```python
from build123d import *

# Parameters (mm, degrees)
SKETCH1_R               = 40
BOSS_EXTRUDE1_DEPTH     = 31.5
CUT_EXTRUDE1_DEPTH      = 65.747586828
CUT_EXTRUDE1_DEPTH_BACK = 65.747586828
SKETCH2_R               = 3
SKETCH7_R               = 10
CUT_EXTRUDE3_DEPTH      = 21
SKETCH8_R               = 6.5
CUT_EXTRUDE4_DEPTH      = 8
SKETCH9_R               = 7.5
CUT_EXTRUDE5_DEPTH      = 6
SKETCH10_R              = 2
CUT_EXTRUDE7_DEPTH      = 65.747587
CIRPATTERN1_COUNT       = 4
SKETCH12_R              = 4
CUT_EXTRUDE8_DEPTH      = 4
CIRPATTERN2_COUNT       = 4
FILLET1_R               = 4


with BuildPart() as part:
    # Sketch1 → Boss-Extrude1 (new body)
    with BuildSketch(Plane(origin=(0, 0, 0), x_dir=(1, 0, 0), z_dir=(0, 1, 0))):
        with Locations(Location((0, 0, 0), (0, 0, 270))):
            Circle(SKETCH1_R)
    extrude(amount=BOSS_EXTRUDE1_DEPTH)

    # Sketch2 → Cut-Extrude1 (cut, two sides: drawn at the far end of the back side and taken through both)
    with BuildSketch(Plane.XY.offset(-CUT_EXTRUDE1_DEPTH_BACK)):
        with Locations((0, 12.5)):
            Circle(SKETCH2_R)
    extrude(amount=CUT_EXTRUDE1_DEPTH + CUT_EXTRUDE1_DEPTH_BACK, mode=Mode.SUBTRACT)

    # Sketch7 → Cut-Extrude3 (cut)
    with BuildSketch(Plane.XZ):
        with Locations(Location((0, 0, 0), (0, 0, 270))):
            Circle(SKETCH7_R)
    extrude(amount=-CUT_EXTRUDE3_DEPTH, mode=Mode.SUBTRACT)

    # Sketch8 → Cut-Extrude4 (cut)
    with BuildSketch(Plane.XY.offset(40)):
        with Locations((0, 12.5)):
            Circle(SKETCH8_R)
    extrude(amount=-CUT_EXTRUDE4_DEPTH, mode=Mode.SUBTRACT)

    # Sketch9 → Cut-Extrude5 (cut)
    with BuildSketch(Plane(origin=(0, 0, -40), x_dir=(-1, 0, 0), z_dir=(0, 0, -1))):
        with Locations((0, 12.5)):
            Circle(SKETCH9_R)
    extrude(amount=-CUT_EXTRUDE5_DEPTH, mode=Mode.SUBTRACT)

    # Sketch10 → Cut-Extrude7 (cut, symmetric)
    with BuildSketch(Plane(origin=(0, 31.5, 0), x_dir=(1, 0, 0), z_dir=(0, 1, 0))):
        with Locations(Location((-19.774516002, -19.823894806, 0), (0, 0, 270))):
            Circle(SKETCH10_R)
    cut_extrude7 = extrude(amount=CUT_EXTRUDE7_DEPTH, both=True, mode=Mode.SUBTRACT)

    # CirPattern1: Cut-Extrude7 ×4 about axis
    cirpattern1_axis = Axis((0, 0, 0), (0, 1, 0))
    for i in range(1, CIRPATTERN1_COUNT):
        add(cut_extrude7.rotate(cirpattern1_axis, i * 360 / CIRPATTERN1_COUNT), mode=Mode.SUBTRACT)

    # Sketch12 → Cut-Extrude8 (cut)
    with BuildSketch(Plane(origin=(0, 0, 0), x_dir=(-1, 0, 0), z_dir=(0, -1, 0))):
        with Locations(Location((-19.774516002, 19.823894806, 0), (0, 0, 90))):
            Circle(SKETCH12_R)
    cut_extrude8 = extrude(amount=-CUT_EXTRUDE8_DEPTH, mode=Mode.SUBTRACT)

    # CirPattern2: Cut-Extrude8 ×4 about axis
    cirpattern2_axis = Axis((0, 0, 0), (0, 1, 0))
    for i in range(1, CIRPATTERN2_COUNT):
        add(cut_extrude8.rotate(cirpattern2_axis, i * 360 / CIRPATTERN2_COUNT), mode=Mode.SUBTRACT)

    # Fillet1
    fillet1_edges = [part.edges().sort_by_distance(p)[0] for p in [
        (0, 0, -40),
    ]]
    fillet(fillet1_edges, radius=FILLET1_R)


solid = part.part
```
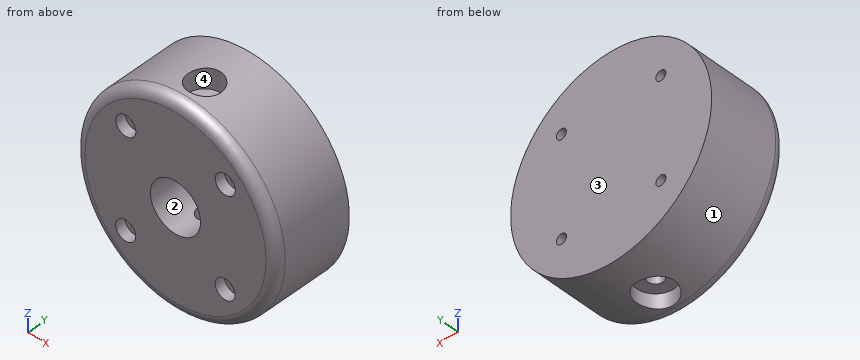
Work out the finished part from the listing and answer in its coordinate system (mm). Face numbers are marked on the shaded views. Give positions to 0.01 mm unless a question says otherwise; leave off trailing zeros. Loops run counter-clockwise (first coordinate to the right, second up) from the corner with the lowest first, then second, coordinate; pieces in that order, holes last. Notation, with made-up numbers: M -26,37.5 L 8,37.5 A33 ccw 8,65.5 Z; hole C -7,69 d7. An arc over 180 degrees is marked long. One line per item, written item: value. Start each with the question number.
1. Each of these flat-tipped pins is pushed along its axis until it touches: P1, Ø12, axis at x = 23, z = -5.5, coming from the -Y side; P2, Ø5, axis at x = 7.5, y = 19, coming from the -Z side; P3, Ø2, axis at x = 19.5, y = 13.5, coming from the +Z side; P4, Ø5, axis at x = 19.82, z = 19.77, coming from the -Y side. Where does it stop, or does it pass through?
2. Determine the mould class of the marked faces 1, 2, 3 and 4 for opening direction X: released by +X, released by -X, zero draft, split by the parting line, or undercut.
3. Find section A-A (y = 13.5). Give the vertices of the cut face in (x, z).
4. Find section B-B (z = 0). Give the vertices of the cut face in (x, y), and give its area (3 significant figures).
5. Find section D-D (y = 8). Give the vertices of the cut face in (x, z).
6. Find the intervals of material crossed by probe 1 along Z at (x, y) = (20.5, 19); probe 2 along X at (y, z) = (12.5, -19.75); probe 3 along Y at (x, z) = (0, 2), in increasing order.
7. Find section C-C (x = 0). Give the vertices of the cut face in (y, z).
Reported:
1. P1: stops at y = 0
1. P2: stops at z = -39.69
1. P3: stops at z = 35.46
1. P4: stops at y = 4
2. face 1: split by the parting line
2. face 2: undercut
2. face 3: zero draft
2. face 4: undercut
3. outline: M -7.43,-39.3 L -7.43,-34 L -2.83,-34 L -2.83,-9.59 A10 cw -2.83,9.59 L -2.83,32 L -6.42,32 L -6.42,39.48 A40 ccw Z; M 2.83,-34 L 7.43,-34 L 7.43,-39.3 A40 ccw 6.42,39.48 L 6.42,32 L 2.83,32 L 2.83,9.59 A10 cw 2.83,-9.59 Z; hole C -19.82,-19.77 d4; hole C -19.77,19.82 d4; hole C 19.77,-19.82 d4; hole C 19.82,19.77 d4
4. outline: M -40,4 A4 ccw -36,0 L -10,0 L -10,21 L 10,21 L 10,0 L 36,0 A4 ccw 40,4 L 40,31.5 L -40,31.5 Z
4. area: 2,090 mm²
5. outline: M -6,-39.55 L -6,-34 L 6,-34 L 6,-39.55 A40 ccw 4.69,39.72 L 4.69,32 L -4.69,32 L -4.69,39.72 A40 ccw Z; hole C -19.82,-19.77 d4; hole C -19.77,19.82 d4; hole C 0,0 d20; hole C 19.77,-19.82 d4; hole C 19.82,19.77 d4
6. probe 1: z = -34.35 to -21.69, -17.96 to 17.89, 21.66 to 34.35
6. probe 2: x = -34.78 to -21.82, -17.82 to -3, 3 to 17.78, 21.77 to 34.78
6. probe 3: y = 21 to 31.5
7. outline: M 0,-36 A4 ccw 4,-40 L 5,-40 L 5,-34 L 9.5,-34 L 9.5,-10 L 0,-10 Z; M 0,10 L 9.5,10 L 9.5,32 L 6,32 L 6,40 L 4,40 A4 ccw 0,36 Z; M 15.5,-34 L 20,-34 L 20,-40 L 31.5,-40 L 31.5,40 L 19,40 L 19,32 L 15.5,32 L 15.5,10 L 21,10 L 21,-10 L 15.5,-10 Z
